from build123d import *

# Parameters (mm, degrees)
SKETCH2_W           = 25.4
SKETCH2_H           = 400.05
BOSS_EXTRUDE1_DEPTH = 6.35
SKETCH4_W           = 6.35
SKETCH4_H           = 400.05
BOSS_EXTRUDE2_DEPTH = 31.75
SKETCH10_W          = 6.35
SKETCH10_H          = 25.4
BOSS_EXTRUDE6_DEPTH = 19.05
SKETCH12_R          = 4.572
CUT_EXTRUDE3_DEPTH  = 19.05
SKETCH14_W          = 6.35
SKETCH14_H          = 25.4
BOSS_EXTRUDE7_DEPTH = 19.05
SKETCH15_R          = 4.572
CUT_EXTRUDE4_DEPTH  = 19.05
SKETCH16_W          = 353.518259368
SKETCH16_H          = 6.201883549
BOSS_EXTRUDE8_DEPTH = 19.05


with BuildPart() as part:
    # Sketch2 → Boss-Extrude1 (new body)
    with BuildSketch(Plane(origin=(0, 0, 0), x_dir=(1, 0, 0), z_dir=(0, 1, 0))):
        with Locations((12.7, 200.025)):
            Rectangle(SKETCH2_W, SKETCH2_H)
    extrude(amount=BOSS_EXTRUDE1_DEPTH)

    # Sketch4 → Boss-Extrude2 (add)
    with BuildSketch(Plane(origin=(0, 6.35, 0), x_dir=(1, 0, 0), z_dir=(0, 1, 0))):
        with Locations((22.225, 200.025)):
            Rectangle(SKETCH4_W, SKETCH4_H)
    extrude(amount=BOSS_EXTRUDE2_DEPTH)

    # Sketch10 → Boss-Extrude6 (add)
    with BuildSketch(Plane.ZY.offset(-19.05)):
        with Locations((-396.875, 19.198116451)):
            Rectangle(SKETCH10_W, SKETCH10_H)
    extrude(amount=BOSS_EXTRUDE6_DEPTH)

    # Sketch12 → Cut-Extrude3 (cut)
    with BuildSketch(Plane.XY.offset(-393.7)):
        with Locations((12.7, 19.198116451)):
            Circle(SKETCH12_R)
    extrude(amount=-CUT_EXTRUDE3_DEPTH, mode=Mode.SUBTRACT)

    # Sketch14 → Boss-Extrude7 (add)
    with BuildSketch(Plane.ZY.offset(-19.05)):
        with Locations((-263.525, 19.05)):
            Rectangle(SKETCH14_W, SKETCH14_H)
    extrude(amount=BOSS_EXTRUDE7_DEPTH)

    # Sketch15 → Cut-Extrude4 (cut)
    with BuildSketch(Plane.XY.offset(-260.35)):
        with Locations((12.7, 19.05)):
            Circle(SKETCH15_R)
    extrude(amount=-CUT_EXTRUDE4_DEPTH, mode=Mode.SUBTRACT)

    # Sketch16 → Boss-Extrude8 (add)
    with BuildSketch(Plane.ZY.offset(-19.05)):
        with Locations((-223.290870316, 34.999058226)):
            Rectangle(SKETCH16_W, SKETCH16_H)
    extrude(amount=BOSS_EXTRUDE8_DEPTH)


solid = part.part
Part model, mm, in its own coordinate system. A direction names the side the tool comes from. Coordinates: 2 decimals unless noted, no trailing zeros. Order: outer loops, then holes, each group sorted by start corner. A loop starts at its lowest first (then second) coordinate and runs counter-clockwise, first axis right, second up. Notation, with made-up numbers: M -19,-37 L -14,-37 A26 cw -14,-23 Z; hole C 75.5,49 d11. An arc over 180 degrees is marked long. Use a Markdown table: item, result.
(1) Probe L1, parallel to Z at x = 2.5, y = 11.5; L2, parallel to Y at x = 6.5, z = -278. List the from-to ranges inside material, lowest first.
A:
| item | result |
|---|---|
| L1 | z = -400.05 to -393.7, -266.7 to -260.35 |
| L2 | y = 0 to 6.35, 31.9 to 38.1 |
(2) Cut at C-C on z = -34.5. Write the cut outline in (x, y), then the cut area to 3 significant figures.
A:
| item | result |
|---|---|
| outline | M 0,0 L 25.4,0 L 25.4,38.1 L 19.05,38.1 L 19.05,6.35 L 0,6.35 Z |
| area | 363 mm^2 |
(3) Cut at B-B on z = -222.5. Write the cut outline in (x, y), then the cut area to 3 significant figures.
A:
| item | result |
|---|---|
| outline | M 0,0 L 25.4,0 L 25.4,38.1 L 0,38.1 L 0,31.9 L 19.05,31.9 L 19.05,6.35 L 0,6.35 Z |
| area | 481 mm^2 |
(4) Cut at A-A on x = 3.5. Write the cut outline in (y, z).
A:
| item | result |
|---|---|
| outline | M 0,-400.05 L 6.35,-400.05 L 6.35,-266.7 L 31.75,-266.7 L 31.75,-260.35 L 6.35,-260.35 L 6.35,0 L 0,0 Z; M 6.5,-400.05 L 38.1,-400.05 L 38.1,-46.53 L 31.9,-46.53 L 31.9,-393.7 L 6.5,-393.7 Z |
(5) Pull direction Y, two halves, no side cores. Call faces 5 (the flat face through (10, 15, -400.05)), 6 (the flat face through (13, 38.1, -203)), 7 (the flat face through (10, 31.898, -223)): released by +Y, released by -Y, zero draft, split by the parting line, or undercut.
A:
| item | result |
|---|---|
| face 5 | zero draft |
| face 6 | released by +Y |
| face 7 | undercut |
(6) Flat gauge pins, fed straight in: pin 1 (1.5 mm diameter, centred on x = 3.5, y = 27.5, fed in from +Z); pin 2 (5 mm diameter, centred on x = 10, y = 36, fed in from +Z); pin 3 (9.5 mm diameter, centred on x = 14, y = 18, fed in from +Z); pin 4 (5.5 mm diameter, centred on x = 12.7, y = 19.05, fed in from +Z). Where does each tip first touch, or does it go through?
A:
| item | result |
|---|---|
| pin 1 | stops at z = -260.35 |
| pin 2 | stops at z = -46.53 |
| pin 3 | stops at z = -260.35 |
| pin 4 | passes through |
(7) Tool access for faces 1 (the flat face through (21, 10, 0)), 2 (the flat face through (9, 6.35, -132)), 3 (the flat face through (10, 35, -46.532)), 4 (the flat face through (7.5, 19, -393.7)): list every direction of +Z, -Z, +X, -X, +Y, -Y with a clear straight run to the whole face (end or side of a thin tool).
A:
| item | result |
|---|---|
| face 1 | +Z, +X, -X, +Y, -Y |
| face 2 | +Z, -X |
| face 3 | +Z, -X, +Y |
| face 4 | -X |
